from build123d import *

# Parameters (mm, degrees)
SKETCH1_W           = 59.5
SKETCH1_H           = 50
SKETCH1_R           = 3
BOSS_EXTRUDE1_DEPTH = 1.5
BOSS_EXTRUDE2_DEPTH = 50
CUT_EXTRUDE1_DEPTH  = 2
CHAMFER1_SIZE       = 2


with BuildPart() as part:
    # Sketch1 → Boss-Extrude1 (new body)
    with BuildSketch(Plane(origin=(0, 0, 0), x_dir=(1, 0, 0), z_dir=(0, 1, 0))):
        Rectangle(SKETCH1_W, SKETCH1_H)
        with Locations(Location((0, 0, 0), (0, 0, 270))):
            Circle(SKETCH1_R, mode=Mode.SUBTRACT)
    extrude(amount=BOSS_EXTRUDE1_DEPTH)

    # Sketch2 → Boss-Extrude2 (add)
    with BuildSketch(Plane(origin=(0, 0, -25), x_dir=(-1, 0, 0), z_dir=(0, 0, -1))):
        Polygon((-29.75, 1.5), (29.75, 1.5), (29.75, 2.5), (28.56, 4), (27.37, 2.5), (26.18, 4), (24.99, 2.5), (23.8, 4), (22.61, 2.5), (21.42, 4), (20.23, 2.5), (19.04, 4), (17.85, 2.5), (16.66, 4), (15.47, 2.5), (14.28, 4), (13.09, 2.5), (11.9, 4), (10.71, 2.5), (9.52, 4), (8.33, 2.5), (7.14, 4), (5.95, 2.5), (4.76, 4), (3.57, 2.5), (2.38, 4), (1.19, 2.5), (0, 4), (-1.19, 2.5), (-2.38, 4), (-3.57, 2.5), (-4.76, 4), (-5.95, 2.5), (-7.14, 4), (-8.33, 2.5), (-9.52, 4), (-10.71, 2.5), (-11.9, 4), (-13.09, 2.5), (-14.28, 4), (-15.47, 2.5), (-16.66, 4), (-17.85, 2.5), (-19.04, 4), (-20.23, 2.5), (-21.42, 4), (-22.61, 2.5), (-23.8, 4), (-24.99, 2.5), (-26.18, 4), (-27.37, 2.5), (-28.56, 4), (-29.75, 2.5), align=None)
    extrude(amount=-BOSS_EXTRUDE2_DEPTH)

    # Sketch3 → Cut-Extrude1 (cut)
    with BuildSketch(Plane(origin=(0, 0, 0), x_dir=(-1, 0, 0), z_dir=(0, -1, 0))):
        with BuildLine():
            Line((-1.75, -2.436698586), (-1.75, -5))
            Line((-1.75, -5), (1.75, -5))
            Line((1.75, -5), (1.75, -2.436698586))
            ThreePointArc((1.75, -2.436698586), (0, 3), (-1.75, -2.436698586))
        make_face()
    extrude(amount=-CUT_EXTRUDE1_DEPTH, mode=Mode.SUBTRACT)

    # Chamfer1
    chamfer1_edges = [part.edges().sort_by_distance(p)[0] for p in [
        (0, 0, 5),
    ]]
    chamfer(chamfer1_edges, length=CHAMFER1_SIZE - 0.0001)  # a hair under: the kernel refuses the full size


solid = part.part
Work out the finished part from the listing and answer in its coordinate system (mm). A direction names the side the tool comes from. Round coordinates to 2 decimals unless told otherwise and drop trailing zeros. Put each result on its own line as item: value. Start each with the question number.
Q1. For a pull along X with two mould halves and no side action, classify faces 3 (the flat face through (-24.403, 3.24, -0.35)), 4 (the flat face through (0, 2, 25)), 5 (the flat face through (29.75, 1, 0)) as pulls with the +X half, pulls with the -X half, needs draft (parallel to the pull), parting line crosses it, or undercut.
Q2. Flat-ended cylindrical pins translate along their axes: pin 1 (3.5 mm diameter, centred on x = 0, z = 0, fed in from +Y); pin 2 (4 mm diameter, centred on x = 8.5, z = 3, fed in from -Y); pin 3 (1.8 mm diameter, centred on x = 0, z = 1, fed in from -Y). Find the tip coordinate at first contact, or state that the pin passes through.
Q3. Straight lines are drawn through the part: L1, parallel to X at y = 1.9, z = 0; L2, parallel to X at y = 1.5, z = 2.5; L3, parallel to Z at x = 0, y = 1.05. For each, find the intervals that lie inside material, in ascending order. Write a range as [from, to].
Q4. A tool of negligible diameter and unlimited length cuts with its end or side. For faces 1 (the flat face through (1.75, 1, 4)), 2 (the flat face through (-4.173, 3.26, -0.35)), from which of +Z, -Z, +X, -X, +Y, -Y can it reach the whole face along a straight path? Write none if from no direction.
Q5. Section A-A, the plane y = 3.35 is taken. Give the number of separate pieces and of enclosed holes in the cut face, and give its area (3 significant figures).
Findings below:
1. face 3: undercut
1. face 4: needs draft
1. face 5: pulls with the +X half
2. pin 1: stops at y = 4
2. pin 2: stops at y = 0
2. pin 3: stops at y = 2
3. L1: x = [-29.75, -3], [3, 29.75]
3. L2: x = [-29.75, -1.75], [1.75, 29.75]
3. L3: z = [-25, -3], [5.95, 25]
4. face 1: -Y
4. face 2: +Z, -Z, +Y
5. separate pieces: 25
5. enclosed holes: 0
5. area: 1,290 mm^2
